Could you check a few things on this drawing? It's one solid part, dimensions in mm from its lowest x, y, z. Round coordinates to 2 decimals unless told otherwise and drop trailing zeros. Loops run counter-clockwise (first coordinate to the right, second up) from the corner with the lowest first, then second, coordinate; pieces in that order, holes last. Notation, with made-up numbers: (55, -38.75) -> (62, -38.75) arc R20 cw to (62, -3.75) -> close; hole circle Ø4 at (-39.75, -24). An arc over 180 degrees is marked (long way). Use one line per item in the form item = value. Start each with the question number.
Item 1: If I drill on L1, parallel to X at y = 1.5, z = 275; L2, parallel to Z at x = 90, y = 0.95 (1 decimal); L3, parallel to Z at x = 50, y = 0.85 (1 decimal), over which ranges is the centre line in solid material (lowest first)? Write a range as [from, to].
Item 2: If we section it at A-A (y = 0.45): Write out the boundary of the cut face in (x, z) (1 decimal), then the cut area to 3 significant figures.
Item 3: I'm going to push a flat-ended pin straight in: pin 1 Ø2.5 at (x, z) = (50, 275) entering from -Y (3 decimals). Where does the tip first touch, or does it pass through?
Item 4: If we section it at B-B (x = 26.5): Write out the boundary of the cut face in (y, z) (1 decimal).
Item 5: If we section it at D-D (x = 127.5): Write out the boundary of the cut face in (y, z).
Item 6: If we section it at C-C (z = 255): Write out the boundary of the cut face in (x, y).
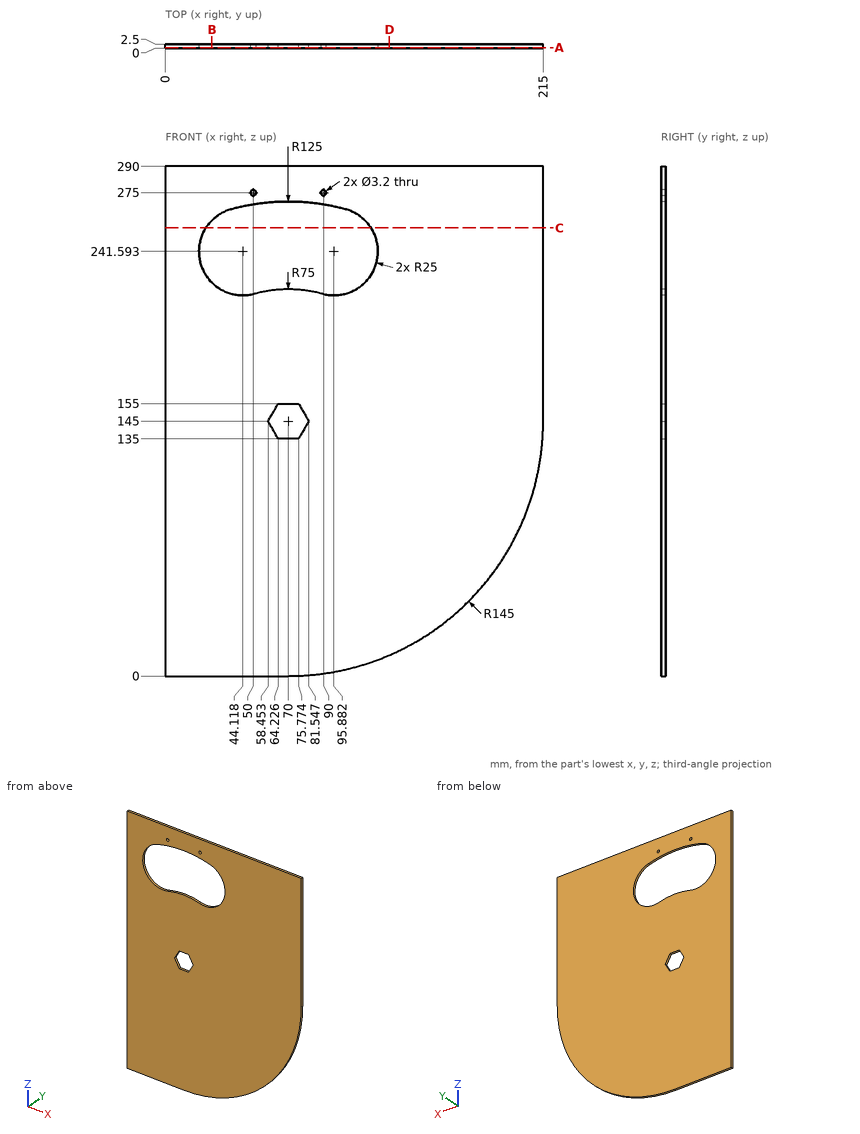
Values found:
q1.L1 = [0, 48.4], [51.6, 88.4], [91.6, 215]
q1.L2 = [1.4, 217.3], [268.4, 273.4], [276.6, 290]
q1.L3 = [0, 217.3], [268.4, 273.4], [276.6, 290]
q2.outline = (0, 0) -> (70, 0) arc R145 ccw to (215, 145) -> (215, 290) -> (0, 290) -> close; hole (37.6, 265.7) arc R25 ccw to (50.6, 217.4) arc R75 cw to (89.4, 217.4) arc R25 ccw to (102.4, 265.7) arc R125 ccw to start; hole circle Ø3.2 at (50, 275); hole (58.5, 145) -> (64.2, 135) -> (75.8, 135) -> (81.5, 145) -> (75.8, 155) -> (64.2, 155) -> close; hole circle Ø3.2 at (90, 275)
q2.area = 52,900 mm2
q3.pin_1 = through
q4.outline = (0, 0) -> (2.5, 0) -> (2.5, 223.9) -> (0, 223.9) -> close; (0, 259.3) -> (2.5, 259.3) -> (2.5, 290) -> (0, 290) -> close
q5.outline = (0, 11.89) -> (2.5, 11.89) -> (2.5, 290) -> (0, 290) -> close
q6.outline = (0, 0) -> (23.02, 0) -> (23.02, 2.5) -> (0, 2.5) -> close; (116.98, 0) -> (215, 0) -> (215, 2.5) -> (116.98, 2.5) -> close
